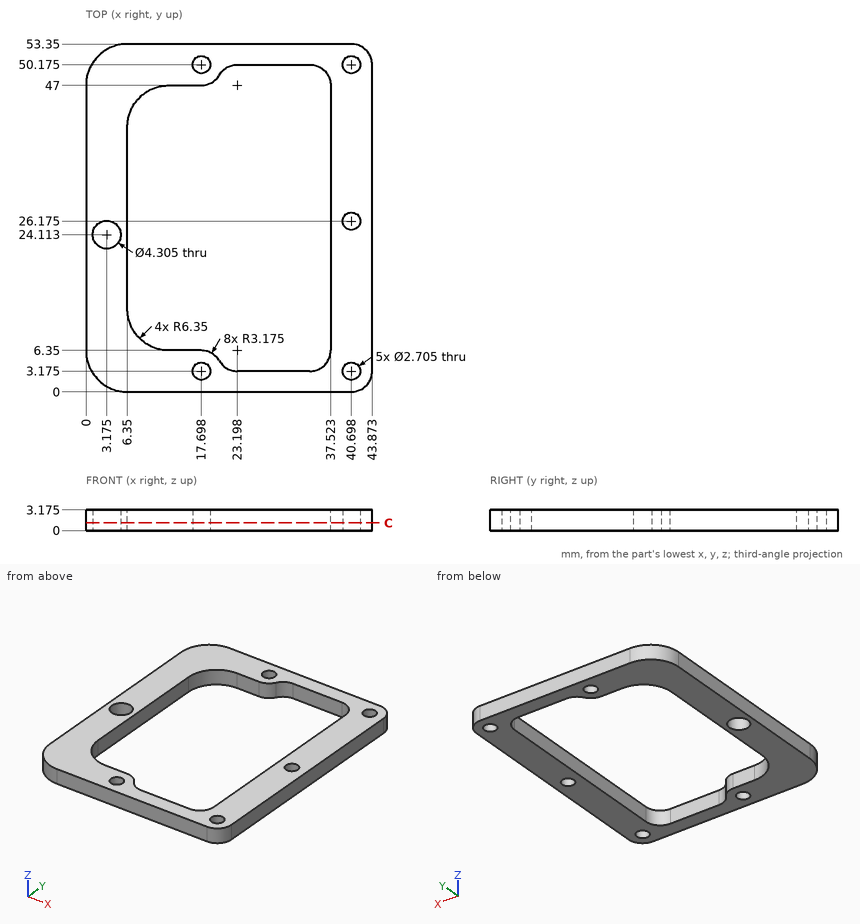
Job drawing, mm, ordinate dimensions from the low corner. One solid piece. Give positions to 0.01 mm unless a question says otherwise; leave off trailing zeros. Return JSON: item names as keys, results as strings.
1) Cut at C-C, the plane z = 1.2. Count the separate pieces of the cut face and the enclosed holes in it.
Geometry says:
{"separate pieces": "1", "enclosed holes": "7"}
2) Flat gauge pin, fed straight in: P1, Ø1.6, axis at y = 32.5, z = 2, coming from the -X side. Where does the tip first touch, or does it go through?
Geometry says:
{"P1": "x = 0"}
3) Probe line 1 (Y direction, x = 40.5, z = 2.9); line 2 (X direction, y = 13.5, z = 2.9); line 3 (Y direction, x = 14.5, z = 1.85). List the from-to ranges inside material, lowest first. Write a range as from..to.
Geometry says:
{"line 1": "0..1.84, 4.51..24.84, 27.51..48.84, 51.51..53.35", "line 2": "0..6.35, 37.52..43.87", "line 3": "0..6.35, 47..53.35"}
